The listing builds one solid part. Answer for the finished solid, in the listing's coordinates (mm). A direction names the side the tool comes from. Coordinates: 2 decimals unless noted, no trailing zeros. Write each loop counter-clockwise with the first axis right and the second up, starting at its lowest first coordinate (ties: lowest second). Pieces come first, ordered by that corner, then holes. Notation, with made-up numbers: M 13,-28.5 L 58,-28.5 A16 cw 58,-13.5 Z; hole C -27,-40 d5. An arc over 180 degrees is marked long. Answer as a JSON object with one key per item and string values. Group by question number.
from build123d import *

# Parameters (mm, degrees)
F0_W     = 127
F0_H     = 127
F0_W_2   = 120.65
F0_H_2   = 120.65
F1_DEPTH = 660.4
F2_R     = 3.175
F3_R     = 3.175
F4_W     = 107.95
F4_H     = 381
F5_DEPTH = 25.4
F6_R     = 7.14375
F7_DEPTH = 25.4
F8_R     = 9.525
F9_DEPTH = 25.4


with BuildPart() as f1:
    # F0 (on Top) → F1 (new body)
    with BuildSketch(Plane.XY):
        Rectangle(F0_W, F0_H)
        Rectangle(F0_W_2, F0_H_2, mode=Mode.SUBTRACT)
    extrude(amount=F1_DEPTH)

    # F2
    f2_edges = [f1.edges().sort_by_distance(p)[0] for p in [
        (60.325, 60.325, 330.2),
        (63.5, -63.5, 330.2),
        (-63.5, -63.5, 330.2),
        (-63.5, 63.5, 330.2),
        (60.325, -60.325, 330.2),
        (63.5, 63.5, 330.2),
        (-60.325, -60.325, 330.2),
    ]]
    fillet(f2_edges, radius=F2_R)

    # F3
    f3_edges = [f1.edges().sort_by_distance(p)[0] for p in [
        (-60.325, 60.325, 330.2),
    ]]
    fillet(f3_edges, radius=F3_R)

    # F4 (on face) → F5 (cut)
    with BuildSketch(Plane.XZ.offset(63.5)):
        with Locations((0, 330.2)):
            Rectangle(F4_W, F4_H)
    extrude(amount=-F5_DEPTH, mode=Mode.SUBTRACT)

    # F6 (on face) → F7 (cut)
    with BuildSketch(Plane.XZ.offset(63.5)):
        with Locations((0, 82.55)):
            Circle(F6_R)
        with Locations((0, 577.85)):
            Circle(F6_R)
    extrude(amount=-F7_DEPTH, mode=Mode.SUBTRACT)

    # F8 (on face) → F9 (cut)
    with BuildSketch(Plane(origin=(0, 63.5, 0), x_dir=(-1, 0, 0), z_dir=(0, 1, 0))):
        with Locations((0, 177.8)):
            Circle(F8_R)
        with Locations((0, 330.2)):
            Circle(F8_R)
        with Locations((0, 482.6)):
            Circle(F8_R)
    extrude(amount=-F9_DEPTH, mode=Mode.SUBTRACT)


solid = f1.part
Item 1: A tool of negligible diameter and unlimited length cuts with its end or side. For faces 4 (the face through (-14, 63.5, 326)), 5 (the face through (-1.549, -61.935, 570.876)), 6 (the face through (12, 60.325, 326)), from which of +Z, -Z, +X, -X, +Y, -Y can it reach the whole face along a straight path? Write none if from no direction.
Item 2: A cutting plane is placed at A-A, the plane x = 37. Write down the section's boundary in (y, z) (3 decimals).
Item 3: Consider L1, parallel to Z at x = 0, y = 61 (3 decimals); L2, parallel to X at y = -16, z = 321 (3 decimals). Determine where each line is inside the solid, lowest interval first. Write a range as from..to.
Item 4: A cutting plane is placed at C-C, the plane x = 0. State how many separate pieces and enclosed holes the cut face has, and give its area (3 significant figures).
Item 5: A cutting plane is placed at B-B, the plane y = 22.5. Write down the section's boundary in (x, z) (3 decimals), and give its area (3 significant figures).
Item 6: A cutting plane is placed at D-D, the plane z = 368.5. Write down the section's boundary in (x, y) (3 decimals).
Item 7: Flat-ended cylindrical pins translate along their axes: pin 1 Ø1.6 at (y, z) = (-62.5, 332) entering from +X; pin 2 Ø17 at (x, z) = (0, 482.6) entering from -Y; pin 3 Ø16.5 at (x, z) = (0, 577.85) entering from -Y; pin 4 Ø2 at (x, z) = (-29.5, 517) entering from -Y (3 decimals). Find the tip coordinate at first contact, or state that the pin passes through.
Item 8: For a pull along Z with two mould halves and no side action, classify faces 1 (the face through (2.06, 61.93, 320.9)), 2 (the face through (60.325, -1, 326)), 3 (the face through (-5, -61, 0)) as +Z half, -Z half, draft (parallel to the pull), parting line (faces both ways), or undercut.
Answer:
{
 "1": {"face 4": "+Z, -Z, +X, -X, +Y", "face 5": "-Y", "face 6": "+Z, -Z"},
 "2": {"outline": "M -63.5,0 L -60.325,0 L -60.325,139.7 L -63.5,139.7 Z; M -63.5,520.7 L -60.325,520.7 L -60.325,660.4 L -63.5,660.4 Z; M 60.325,0 L 63.5,0 L 63.5,660.4 L 60.325,660.4 Z"},
 "3": {"L1": "0..168.275, 187.325..320.675, 339.725..473.075, 492.125..660.4", "L2": "-63.5..-60.325, 60.325..63.5"},
 "4": {"separate pieces": "8", "enclosed holes": "0", "area": "2,710 mm2"},
 "5": {"outline": "M -63.5,0 L -60.325,0 L -60.325,660.4 L -63.5,660.4 Z; M 60.325,0 L 63.5,0 L 63.5,660.4 L 60.325,660.4 Z", "area": "4,190 mm2"},
 "6": {"outline": "M -63.5,-60.325 A3.175 ccw -60.325,-63.5 L -53.975,-63.5 L -53.975,-60.325 L -57.15,-60.325 A3.175 cw -60.325,-57.15 L -60.325,57.15 A3.175 cw -57.15,60.325 L 57.15,60.325 A3.175 cw 60.325,57.15 L 60.325,-57.15 A3.175 cw 57.15,-60.325 L 53.975,-60.325 L 53.975,-63.5 L 60.325,-63.5 A3.175 ccw 63.5,-60.325 L 63.5,60.325 A3.175 ccw 60.325,63.5 L -60.325,63.5 A3.175 ccw -63.5,60.325 Z"},
 "7": {"pin 1": "x = 63.19", "pin 2": "through", "pin 3": "y = -63.5", "pin 4": "y = 60.325"},
 "8": {"face 1": "undercut", "face 2": "draft", "face 3": "-Z half"}
}
